Design review of the part built by this model. Coordinates are the model's own, in mm. Face numbers are marked on the shaded views. A direction names the side the tool comes from. Round coordinates to 2 decimals unless told otherwise and drop trailing zeros. Write each loop counter-clockwise with the first axis right and the second up, starting at its lowest first coordinate (ties: lowest second). Pieces come first, ordered by that corner, then holes.
from build123d import *

# Parameters (mm, degrees)
F1_DEPTH = 12.5
F2_R     = 4.15
F3_DEPTH = 8
F4_R     = 2


with BuildPart() as f1:
    # F0 (on Right) → F1 (new body, symmetric)
    with BuildSketch(Plane.YZ):
        Polygon((0, -12.309401), (0, 20.609401), (4, 18.3), (4, 40), (-6, 40), (-34, 40), (-34, 32), (-6, 32), (-6, -24), (4, -24), (4, -10), align=None)
    extrude(amount=F1_DEPTH, both=True)

    # F2 (on face) → F3 (cut, through all)
    with BuildSketch(Plane.XY.offset(40)):
        with Locations((0, -28)):
            Circle(F2_R)
    extrude(amount=-F3_DEPTH, mode=Mode.SUBTRACT)

    # F4
    f4_edges = [f1.edges().sort_by_distance(p)[0] for p in [
        (0, -6, 32),
    ]]
    fillet(f4_edges, radius=F4_R)


solid = f1.part
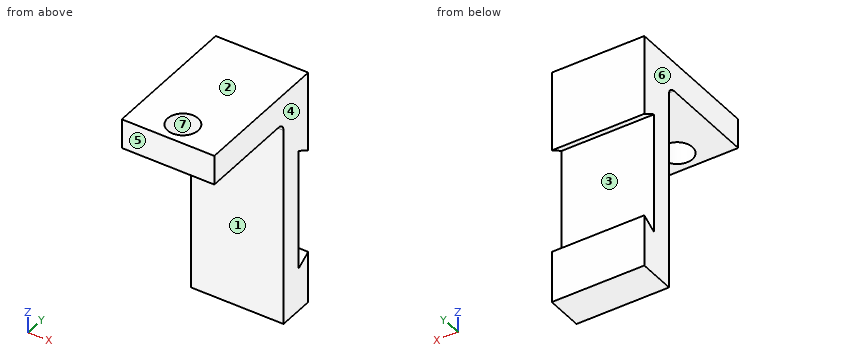
1) Add section D-D on z = 33. State the section outline as (x, y) points, and give its area (3 significant figures).
2) Add section B-B on y = -28. State the section outline as (x, z) points, and give its area (3 significant figures).
3) For the marked faces 1, 2 and 3, list the 3-axis set-ups (+Z, -Z, +X, -X, +Y, -Y) from which the entire face can be reached by the end or side of a thin tool; tool diameter is ignored.
4) For line 1 along Y through (x, z) = (0, 35.25); line 2 along Y through (x, z) = (0.5, -1); line 3 along Y through (x, z) = (6.5, -15.5), list the stretches that pass through material, from the lowest coordinate up.
5) For P1, Ø7.5, axis at x = -5, z = 2, coming from the -Y side; P2, Ø3, axis at x = -7, z = -8, coming from the +Y side; P3, Ø13.5, axis at x = 0, y = -28, coming from the +Z side; P4, Ø6, axis at x = 4.5, y = -27.5, coming from the -Z side, all flat-tipped, find the tip position at first contact; note any pin that passes through.
6) The part is to be moulded in two halves that separate along X. For the marked faces 4, 5, 6 and 7, say which applies: pulls with the +X half, pulls with the -X half, needs draft (parallel to the pull), parting line crosses it, or undercut.
7) Add section A-A on x = 0. State the section outline as (y, z) points.
8) Add section C-C on x = 5.75. State the section outline as (y, z) points.
Computed:
1. outline: (-12.5, -34) - (12.5, -34) - (12.5, 4) - (-12.5, 4) - close; hole circle Ø8.3 at (0, -28)
1. area: 896 mm2
2. outline: (-12.5, 32) - (-4.15, 32) - (-4.15, 40) - (-12.5, 40) - close; (4.15, 32) - (12.5, 32) - (12.5, 40) - (4.15, 40) - close
2. area: 134 mm2
3. face 1: -Z, +X, -X, -Y
3. face 2: +Z, +X, -X, +Y, -Y
3. face 3: +X, -X
4. line 1: y = -34 to -32.15, -23.85 to 4
4. line 2: y = -6 to 0
4. line 3: y = -6 to 4
5. P1: stops at y = -6
5. P2: stops at y = 0
5. P3: stops at z = 40
5. P4: stops at z = 32
6. face 4: pulls with the +X half
6. face 5: needs draft
6. face 6: pulls with the -X half
6. face 7: undercut
7. outline: (-34, 32) - (-32.15, 32) - (-32.15, 40) - (-34, 40) - close; (-23.85, 32) - (-8, 32) arc R2 cw to (-6, 30) - (-6, -24) - (4, -24) - (4, -10) - (0, -12.31) - (0, 20.61) - (4, 18.3) - (4, 40) - (-23.85, 40) - close
8. outline: (-34, 32) - (-8, 32) arc R2 cw to (-6, 30) - (-6, -24) - (4, -24) - (4, -10) - (0, -12.31) - (0, 20.61) - (4, 18.3) - (4, 40) - (-34, 40) - close
